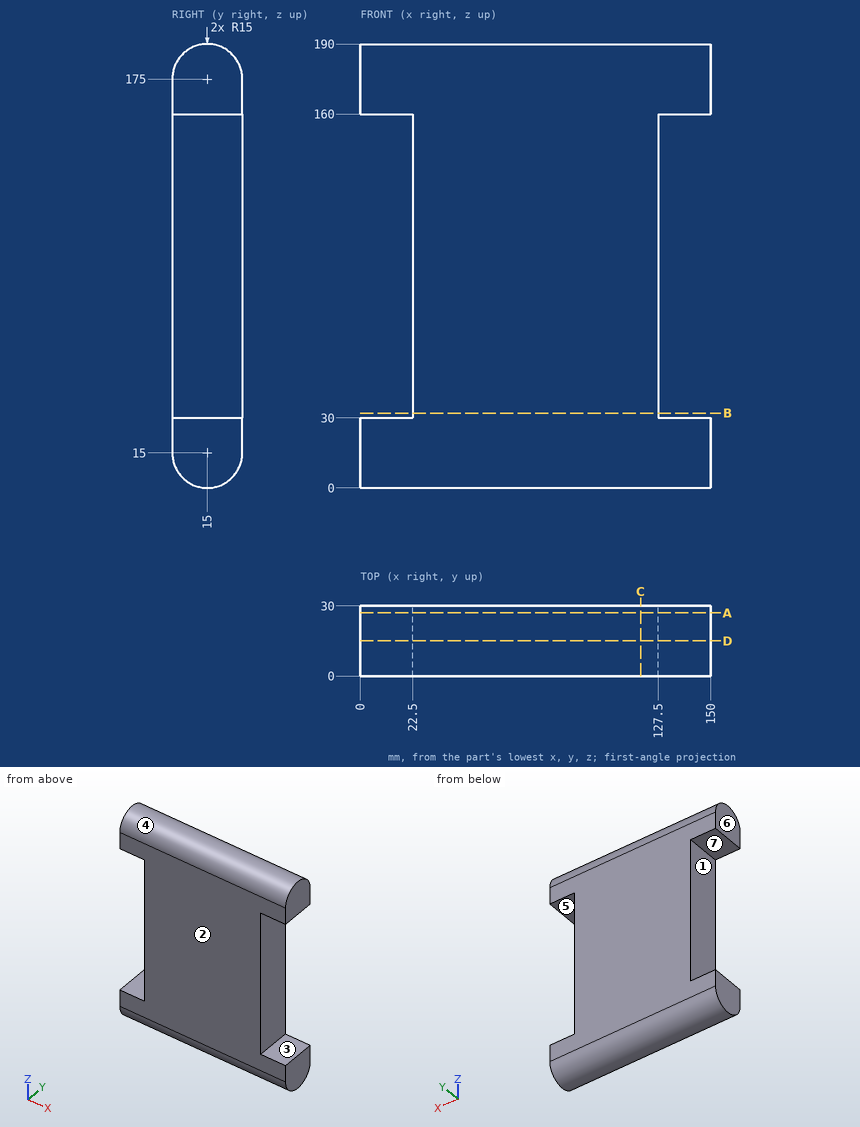
Answer from the drawing. Dimensions are ordinates in mm from the lowest x, y and z of the part. A direction names the side the tool comes from. Round coordinates to 2 decimals unless told otherwise and drop trailing zeros. Write each loop counter-clockwise with the first axis right and the second up, starting at its lowest first coordinate (ties: lowest second). Pieces come first, ordered by that corner, then holes.
1. The part is cut by section D-D, the plane y = 15. Determine the outline of the cut face in (x, z).
2. Which of the six approach directions +Z, -Z, +X, -X, +Y, -Y give full straight-line access (tool end or side, diameter ignored) to the marked faces 1, 2 and 3?
3. Determine the mould class of the marked faces 4, 5, 6 and 7 for opening direction Z: pulls with the +Z half, pulls with the -Z half, needs draft (parallel to the pull), parting line crosses it, or undercut.
4. The part is cut by section C-C, the plane x = 120. Determine the outline of the cut face in (y, z).
5. The part is cut by section B-B, the plane z = 32. Determine the outline of the cut face in (x, y), then the cut area to 3 significant figures.
6. Straight lines are drawn through the part: L1, parallel to Z at x = 135.5, y = 14; L2, parallel to X at y = 23, z = 98; L3, parallel to Z at x = 33.5, y = 2. For each, find the intervals that lie inside material, in ascending order.
7. Given pin 1 Ø4 at (x, y) = (46, 10.5) entering from +Z; pin 2 Ø3 at (y, z) = (7, 123) entering from +X; pin 3 Ø10 at (x, y) = (128.5, 25) entering from -Z, each flat-ended and moving along its own axis, determine where each tip first touches the part or whether it passes through.
8. The part is cut by section A-A, the plane y = 27. Determine the outline of the cut face in (x, z).
Values:
1. outline: (0, 0) - (150, 0) - (150, 30) - (127.5, 30) - (127.5, 160) - (150, 160) - (150, 190) - (0, 190) - (0, 160) - (22.5, 160) - (22.5, 30) - (0, 30) - close
2. face 1: -X, +Y, -Y
2. face 2: +Z, -Z, +X, -X, -Y
2. face 3: +X, +Y, -Y
3. face 4: pulls with the +Z half
3. face 5: undercut
3. face 6: needs draft
3. face 7: undercut
4. outline: (0, 15) arc R15 ccw to (30, 15) - (30, 175) arc R15 ccw to (0, 175) - close
5. outline: (22.5, 0) - (127.5, 0) - (127.5, 30) - (22.5, 30) - close
5. area: 3,150 mm2
6. L1: z = 0.03 to 30, 160 to 189.97
6. L2: x = 22.5 to 127.5
6. L3: z = 7.52 to 182.48
7. pin 1: stops at z = 189.79
7. pin 2: stops at x = 127.5
7. pin 3: stops at z = 0.86
8. outline: (0, 6) - (150, 6) - (150, 30) - (127.5, 30) - (127.5, 160) - (150, 160) - (150, 184) - (0, 184) - (0, 160) - (22.5, 160) - (22.5, 30) - (0, 30) - close
